```python
from build123d import *

# Parameters (mm, degrees)
PAD_DEPTH       = 180
SKETCH001_W     = 29.620193
SKETCH001_H     = 118
POCKET_DEPTH    = 70.001
SKETCH002_W     = 70
SKETCH002_H     = 7.16013
PAD001_DEPTH    = 30
SKETCH003_R     = 15
SKETCH003_R_2   = 7.5
PAD002_DEPTH    = 30
FILLET_R        = 5
FILLET001_R     = 5
SKETCH004_R     = 7.5
POCKET001_DEPTH = 30
PAD003_DEPTH    = 70


with BuildPart() as part:
    # Sketch → Pad (new body)
    with BuildSketch(Plane.XZ):
        Polygon((15, 0), (35, 0), (35, 50), (-35, 50), (-35, 0), (-15, 0), (-15, 20), (-10, 20), (-10, 40), (10, 40), (10, 20), (15, 20), align=None)
    extrude(amount=-PAD_DEPTH)

    # Sketch001 → Pocket (cut, through all)
    with BuildSketch(Plane(origin=(35, 0, 0), x_dir=(0, 0, 1), z_dir=(1, 0, 0))):
        with Locations((49.810097, -91)):
            Rectangle(SKETCH001_W, SKETCH001_H)
    extrude(amount=-POCKET_DEPTH, mode=Mode.SUBTRACT)

    # Sketch002 → Pad001 (new body)
    with BuildSketch(Plane(origin=(0, 180, 0), x_dir=(1, 0, 0), z_dir=(0, 1, 0))):
        with Locations((0, -51.419935)):
            Rectangle(SKETCH002_W, SKETCH002_H)
    extrude(amount=-PAD001_DEPTH)

    # Sketch003 → Pad002 (new body)
    with BuildSketch(Plane.XZ.offset(-150)):
        with Locations((0, 60)):
            Circle(SKETCH003_R)
        with Locations((0, 60)):
            Circle(SKETCH003_R_2, mode=Mode.SUBTRACT)
    extrude(amount=-PAD002_DEPTH)

    # Fillet
    fillet_edges = [part.edges().sort_by_distance(p)[0] for p in [
        (14.142136, 165, 55),
    ]]
    fillet(fillet_edges, radius=FILLET_R)

    # Fillet001
    fillet001_edges = [part.edges().sort_by_distance(p)[0] for p in [
        (-14.142136, 165, 55),
    ]]
    fillet(fillet001_edges, radius=FILLET001_R)

    # Sketch004 → Pocket001 (cut)
    with BuildSketch(Plane(origin=(0, 180, 0), x_dir=(1, 0, 0), z_dir=(0, 1, 0))):
        with Locations((0, -60)):
            Circle(SKETCH004_R)
    extrude(amount=-POCKET001_DEPTH, mode=Mode.SUBTRACT)

    # Sketch005 → Pad003 (new body)
    with BuildSketch(Plane(origin=(35, 0, 0), x_dir=(0, 0, 1), z_dir=(1, 0, 0))):
        with BuildLine():
            Line((50, -32), (80, -32))
            ThreePointArc((80, -32), (70.746374, -12.11514), (50, -5))
            Line((50, -32), (50, -5))
        make_face()
    extrude(amount=-PAD003_DEPTH)


solid = part.part
```
Verification items for the finished model (mm, model axes). A direction names the side the tool comes from. Coordinates: 2 decimals unless noted, no trailing zeros. Order: outer loops, then holes, each group sorted by start corner. A loop starts at its lowest first (then second) coordinate and runs counter-clockwise, first axis right, second up. Notation, with made-up numbers: (-28, -17) -> (9, -17) arc R28 cw to (9, 10) -> close; hole circle Ø8 at (61.5, 55.5). An arc over 180 degrees is marked (long way). Put each result on its own line as item: value. Start each with the question number.
1) Release check for a two-part mould opening along Y. For faces 1 (the cylindrical face through (16, 165, 57)), 2 (the flat face through (0, 32, 57)), 3 (the flat face through (0, 0, 42)) record: pulls with the +Y half, pulls with the -Y half, needs draft (parallel to the pull), parting line crosses it, or undercut.
2) Cross-section at A-A (z = 25.5). Enter the section's corners in (x, y), plus the area to 3 significant figures.
3) Cross-section at B-B (y = 40). Enter the section's corners in (x, z).
4) Tool access check on faces 4 (the flat face through (27, 165, 55)), 5 (the flat face through (0, 150, 51)), 6 (the cylindrical face through (0, 165, 75)), 7 (the flat face through (-15, 89, 10)), 8 (the cylindrical face through (-16, 165, 57)). Record the directions out of +Z, -Z, +X, -X, +Y, -Y that give a thin tool (end or side, any length) a straight path to the whole face; none if there is none.
5) Material ranges on L1, parallel to X at y = 42.5, z = 24; L2, parallel to Z at x = 0, y = 173.5; L3, parallel to Y at x = -10, z = 45, recorded low to high.
6) Cross-section at D-D (x = 22). Enter the section's corners in (y, z).
7) Cross-section at C-C (x = 0). Enter the section's corners in (y, z), plus the area to 3 significant figures.
8) Go/stop test with flat-tipped pins: pin 1 (3 mm diameter, centred on x = 12.5, z = 19.5, fed in from +Y); pin 2 (10 mm diameter, centred on x = 0, y = 9, fed in from -Z); pin 3 (2.5 mm diameter, centred on x = -10.5, y = 2.5, fed in from +Z); pin 4 (4 mm diameter, centred on x = -23, y = 50.5, fed in from +Z). Record where each tip stops, or that it passes through.
Geometry check:
1. face 1: needs draft
1. face 2: undercut
1. face 3: pulls with the -Y half
2. outline: (-35, 0) -> (-10, 0) -> (-10, 180) -> (-35, 180) -> close; (10, 0) -> (35, 0) -> (35, 180) -> (10, 180) -> close
2. area: 9,000 mm^2
3. outline: (-35, 0) -> (-15, 0) -> (-15, 20) -> (-10, 20) -> (-10, 35) -> (-35, 35) -> close; (10, 20) -> (15, 20) -> (15, 0) -> (35, 0) -> (35, 35) -> (10, 35) -> close
4. face 4: +Z, +X, +Y
4. face 5: +Z, +X, -X
4. face 6: +Z, +Y
4. face 7: -Z, +Y, -Y
4. face 8: +Z, -X, +Y
5. L1: x = -35 to -10, 10 to 35
5. L2: z = 40 to 52.5, 67.5 to 75
5. L3: y = 0 to 32, 150 to 180
6. outline: (0, 0) -> (180, 0) -> (180, 55) -> (150, 55) -> (150, 35) -> (32, 35) -> (32, 80) arc R28 ccw to (5, 50) -> (0, 50) -> close
7. outline: (0, 40) -> (32, 40) -> (32, 80) arc R28 ccw to (5, 50) -> (0, 50) -> close; (150, 40) -> (180, 40) -> (180, 52.5) -> (150, 52.5) -> close; (150, 67.5) -> (180, 67.5) -> (180, 75) -> (150, 75) -> close
7. area: 1,560 mm^2
8. pin 1: stops at y = 180
8. pin 2: stops at z = 40
8. pin 3: stops at z = 50
8. pin 4: stops at z = 35
